Autodesk Inventor part; units mm, degrees
ref_plane "YZ Plane" through (0, 0, 0) normal (1, 0, 0) x (0, 1, 0)
ref_plane "XZ Plane" through (0, 0, 0) normal (0, 1, 0) x (-1, 0, 0)
ref_plane "XY Plane" through (0, 0, 0) normal (0, 0, 1) x (1, 0, 0)
sketch "Sketch1" plane through (0, 0, 0) normal (0, 1, 0) x (-1, 0, 0)
  point P0 (0, 0)
sketch "Sketch2" plane through (0, 0, 0) normal (0, 1, 0) x (-1, 0, 0)
  line L0 (68, -12) -> (68, -66)
  line L1 (68, -66) -> (0, -66)
  line L2 (0, -66) -> (0, -12)
  line L3 (68, -12) -> (0, -12)
  point P0 (0, 0)
  dimension "d0" = 68
  dimension "d138" = 54
extrude "Extrusion1" add sketch "Sketch2" along normal blind 17.5
sketch "Sketch3" plane through (0, 17.5, 0) normal (0, 1, 0) x (1, 0, 0)
  line L0 (0, 66) -> (-68, 66)
  line L1 (-68, 66) -> (0, 66)
  line L2 (-68, 66) -> (0, 66)
  line L3 (0, 66) -> (-68, 66)
  line L4 (-68, 66) -> (-68, 12)
  line L5 (-68, 12) -> (0, 12)
  line L6 (0, 66) -> (0, 12)
  dimension "d135" = 68
  dimension "d136" = 54
sketch "Sketch4" plane through (0, 17.5, 0) normal (0, 1, 0) x (1, 0, 0)
  line L0 (0, 66) -> (-68, 66)
  line L1 (-30.4814, 66) -> (-28.4814, 66)
  line L2 (-28.4814, 66) -> (-28.4814, 64)
  line L3 (-68, 66) -> (-68, 12)
  line L4 (-68, 37.8423) -> (-68, 39.8423)
  line L5 (-68, 39.8423) -> (-66, 39.8423)
  line L6 (0, 38.8423) -> (0, 36.8423)
  line L7 (0, 36.8423) -> (-2, 36.8423)
  line L8 (-66, 64) -> (-2, 64)
  line L9 (-2, 64) -> (-2, 14)
  line L10 (-2, 14) -> (-66, 14)
  line L11 (-66, 14) -> (-66, 64)
  dimension "d5" = 2
  dimension "d6" = 2
  dimension "d7" = 2
  dimension "d11" = 2
  dimension "d75" = 2
  dimension "d132" = 50
  dimension "d133" = 64
extrude "Extrusion2" cut sketch "Sketch4" against normal blind 15.5 contours L8 L9 L10 L11
sketch "Sketch7" plane through (0, 17.5, 0) normal (0, 1, 0) x (1, 0, 0)
  line L0 (-68, 66) -> (-67, 66)
  line L1 (-68, 66) -> (-6, 66)
  line L2 (-68, 65) -> (-68, 66)
  line L3 (0, 66) -> (-7, 66)
  line L4 (-67, 65) -> (-1, 65)
  line L5 (0, 66) -> (-68, 66)
  line L6 (-68, 66) -> (0, 66)
  line L7 (0, 12) -> (0, 66)
  line L8 (0, 12) -> (-1, 12)
  line L9 (-1, 66) -> (0, 66)
  line L10 (0, 66) -> (0, 12)
  line L11 (0, 12) -> (-1, 12)
  line L12 (-68, 12) -> (0, 12)
  line L13 (-1, 65) -> (-1, 12)
  line L14 (0, 12) -> (-1, 12)
  line L15 (-67, 65) -> (-67, 12)
  line L16 (-68, 66) -> (-68, 12)
  line L17 (-67, 12) -> (-68, 12)
  line L18 (-68, 12) -> (-68, 66)
  dimension "d76" = 1
  dimension "d139" = 1
  dimension "d140" = 1
extrude "Extrusion3" cut sketch "Sketch7" against normal blind 2 contours L0 L1 L3 L7 L8 L13 L4 L15 L12 L16 L2
sketch "Sketch8" plane through (0, 17.5, 0) normal (0, 1, 0) x (1, 0, 0)
  line L0 (0, 12) -> (0, 13)
  line L1 (0, 13) -> (-68, 13)
  line L2 (0, 12) -> (-68, 12)
  line L3 (-68, 12) -> (-68, 13)
  line L4 (-67, 12) -> (-1, 12)
  point P0 (0, 0)
  point P1 (-70, 0)
  dimension "d46" = 68
  dimension "d141" = 1
extrude "Extrusion4" cut sketch "Sketch8" against normal blind 2
sketch "Sketch10" plane through (0, 2, 0) normal (0, 1, 0) x (1, 0, 0)
  line L0 (-31, 2) -> (-41, 2)
  line L1 (-63, 64) -> (-48, 64)
  line L2 (-48, 64) -> (-48, 61)
  line L3 (-48, 61) -> (-63, 61)
  line L4 (-63, 61) -> (-63, 64)
  line L5 (-22, 14) -> (-7, 14)
  line L6 (-7, 14) -> (-7, 17)
  line L7 (-7, 17) -> (-22, 17)
  line L8 (-22, 17) -> (-22, 14)
  line L9 (-66, 14) -> (-66, 64)
  line L10 (-2, 14) -> (-66, 14)
  line L11 (-66, 64) -> (-2, 64)
  line L12 (-2, 64) -> (-2, 14)
  line L13 (-2, 14) -> (-66, 14)
  line L14 (-66, 14) -> (-66, 64)
  point P0 (0, 0)
  point P1 (-21, 64)
  dimension "d57" = 15
  dimension "d58" = 3
  dimension "d61" = 15
  dimension "d79" = 3
extrude "Extrusion5" add sketch "Sketch10" along normal blind 18 contours L1 L2 L3 L4 | L8 L7 L6 L5
sketch "Sketch11" plane through (0, 0, 0) normal (0, -1, 0) x (1, 0, 0)
  circle A0 centre (-12, -42.73) radius 4
  circle A1 centre (-33.5, -54.23) radius 1.5
  line L0 (0, 0) -> (0, -66)
  line L1 (0, -66) -> (-68, -66)
  line L2 (-2, -64) -> (-2, -14)
  dimension "d85" = 23.27
  dimension "d86" = 21.5
  dimension "d88" = 8
  dimension "d89" = 3
  dimension "d119" = 11.5
  dimension "d120" = 10
extrude "Extrusion6" cut sketch "Sketch11" against normal blind 9
sketch "Sketch12" plane through (0, 0, 0) normal (0, -1, 0) x (1, 0, 0)
  line L0 (-68, -12) -> (-68, -66)
  line L1 (0, -12) -> (0, -6)
  line L2 (0, -6) -> (-68, -6)
  line L3 (-68, -6) -> (-68, -12)
  line L4 (-68, -12) -> (0, -12)
  line L5 (0, -12) -> (-68, -12)
  point P0 (0, 0)
  point P1 (-70, 0)
  dimension "d81" = 6
  dimension "d143" = 68
  dimension "d144" = 0
extrude "Extrusion7" add sketch "Sketch12" against normal blind 29.5
sketch "Sketch15" plane through (0, 0, -66) normal (1, 0, 0) x (0, 0, -1)
  line L0 (-27.77, 17.5) -> (-18.77, 17.5)
  line L1 (-18.77, 17.5) -> (-18.77, 12.5)
  line L2 (-18.77, 12.5) -> (-27.77, 12.5)
  line L3 (-27.77, 12.5) -> (-27.77, 17.5)
  line L4 (-54, 0) -> (-54, 29.5)
  line L5 (0, 0) -> (0, 15.5)
  line L6 (0, 0) -> (-60, 0)
  line L7 (0, 15.5) -> (-54, 15.5)
  line L8 (-23.27, -7.8454) -> (-23.27, 0)
  line L9 (-23.27, 0) -> (-23.27, 15.5)
  point P0 (-66, 0)
  point P1 (-66, 14.75)
  point P2 (0, 16.75)
  dimension "d108" = 9
  dimension "d109" = 5
  dimension "d111" = 27.77
extrude "Extrusion9" cut sketch "Sketch15" against normal blind 10 contours L0 L1 L7 L3 | L7 L9 L2 L3 | L1 L2 L9 L7
fillet "Fillet7" radius 2 1 edges at (0, 7.75, -66)
fillet "Fillet8" radius 2 1 edges at (-68, 7.75, -66)
fillet "Fillet9" radius 2 1 edges at (0, 14.75, -6)
fillet "Fillet11" radius 2 1 edges at (-68, 14.75, -6)
sketch "Sketch16" plane through (-2, 0, -6) normal (0, 0, 1) x (1, 0, 0)
  line L0 (2, 29.5) -> (-66, 29.5)
  line L1 (-32, 29.5) -> (-32, 0)
  line L2 (-46, 2) -> (0, 2)
  line L3 (-66, 0) -> (-66, 15.5)
  line L4 (-66, 15.5) -> (-66, 29.5)
  line L5 (-32, 14.75) -> (-64, 14.75)
  line L6 (-64, 0) -> (-64, 29.5)
  circle A0 centre (-32, 14.75) radius 2.5
  point P0 (2, 0)
  dimension "d148" = 5
extrude "Extrusion10" cut sketch "Sketch16" against normal blind 6 contours A0 L1 | L1 L5 A0 | L1 A0 L5
sketch "Sketch17" plane through (-2, 0, -66) normal (0, 0, -1) x (-1, 0, 0)
  line L0 (3, 20.5) -> (11.5, 20.5)
  line L1 (11.5, 20.5) -> (11.5, 15.5)
  line L2 (11.5, 15.5) -> (3, 15.5)
  line L3 (3, 15.5) -> (3, 20.5)
  line L4 (18.1, 20.5) -> (26.6, 20.5)
  line L5 (26.6, 20.5) -> (26.6, 15.5)
  line L6 (26.6, 15.5) -> (18.1, 15.5)
  line L7 (18.1, 15.5) -> (18.1, 20.5)
  line L8 (66, 0) -> (66, 15.5)
  line L9 (-1, 17.5) -> (65, 17.5)
  line L10 (64, 15.5) -> (0, 15.5)
  line L11 (-2, 15.5) -> (-2, 0)
  dimension "d151" = 8.5
  dimension "d152" = 8.5
  dimension "d153" = 5
  dimension "d157" = 0
  dimension "d158" = 13.5
  dimension "d160" = 28.6
extrude "Extrusion11" cut sketch "Sketch17" against normal blind 10 contours L0 L1 L9 L3 | L9 L1 L2 L3 | L9 L5 L6 L7 | L7 L4 L5 L9
properties part number "Shell 3 top"
Here's how the part is built. I have some questions about the finished solid (model axes, mm). A direction names the side the tool comes from. Round coordinates to 2 decimals unless told otherwise and drop trailing zeros. Order: outer loops, then holes, each group sorted by start corner. A loop starts at its lowest first (then second) coordinate and runs counter-clockwise, first axis right, second up. Notation, with made-up numbers: (-34.75, 35.25) -> (15.25, 35.25) arc R23 cw to (15.25, 48.25) -> close; hole circle Ø1 at (37.25, 54). An arc over 180 degrees is marked (long way). Use a Markdown table: item, result. Add a question column.
(1) Suppose I cut it at A-A, the plane z = -42.73. Please give me the cut outline in (x, y).
(2) Suppose I cut it at C-C, the plane y = 8. Please give me the cut outline in (x, z), and give its area (3 significant figures).
(3) If we mould it in two halves opening along Z, with no side actions, what happens to faces 1 (the face through (-48, 17, -65)), 2 (the face through (-63, 11, -62)), 3 (the face through (-56, 20, -63))? For each: released by +Z, released by -Z, zero draft, split by the parting line, or undercut.
(4) Suppose I cut it at D-D, the plane z = -62. Please give me the cut outline in (x, y), and give its area (3 significant figures).
(5) For pin 1 Ø1.5 at (x, z) = (-58.5, -63) entering from +Y; pin 2 Ø1 at (y, z) = (18.5, -27.5) entering from -X; pin 3 Ø4 at (x, z) = (-57.5, -15) entering from +Y; pin 4 Ø1.1 at (y, z) = (16.5, -64.5) entering from -X, each with a flat end and sliding along its axis, tell me the tip position at first contact or that it passes through.
(6) Suppose I cut it at B-B, the plane x = -12. Please give me the cut outline in (y, z), and give its area (3 significant figures).
(7) I need wall thicknesses on line 1 along X through (y, z) = (8, -14.5); line 2 along Z through (x, y) = (-10.5, 7.5); line 3 along X through (y, z) = (9.5, -62). Which ranges of each line are inside material? Lowest first, please.
(8) For faces 4 (the face through (-1, 12.5, -43)), 5 (the face through (-25, 10, -64)), 6 (the face through (-1.8, 17.5, -56.7)), 7 (the face through (-56, 19, -64)), which set-ups out of +Z, -Z, +X, -X, +Y, -Y let a thin tool reach every point of the face, with its end or its side?
Verdict:
| question | item | result |
|---|---|---|
| 1 | outline | (-68, 0) -> (-16, 0) -> (-16, 2) -> (-66, 2) -> (-66, 17.5) -> (-67, 17.5) -> (-67, 15.5) -> (-68, 15.5) -> close; (-8, 0) -> (0, 0) -> (0, 12.5) -> (-2, 12.5) -> (-2, 2) -> (-8, 2) -> close |
| 2 | outline | (-68, -64) arc R2 ccw to (-66, -66) -> (-2, -66) arc R2 ccw to (0, -64) -> (0, -8) arc R2 ccw to (-2, -6) -> (-66, -6) arc R2 ccw to (-68, -8) -> close; hole (-66, -64) -> (-63, -64) -> (-63, -61) -> (-48, -61) -> (-48, -64) -> (-2, -64) -> (-2, -14) -> (-7, -14) -> (-7, -17) -> (-22, -17) -> (-22, -14) -> (-66, -14) -> close |
| 2 | area | 967 mm2 |
| 3 | face 1 | released by -Z |
| 3 | face 2 | undercut |
| 3 | face 3 | zero draft |
| 4 | outline | (-68, 0) -> (0, 0) -> (0, 15.5) -> (-1, 15.5) -> (-1, 17.5) -> (-2, 17.5) -> (-2, 2) -> (-48, 2) -> (-48, 20) -> (-63, 20) -> (-63, 2) -> (-66, 2) -> (-66, 17.5) -> (-67, 17.5) -> (-67, 15.5) -> (-68, 15.5) -> close |
| 4 | area | 464 mm2 |
| 5 | pin 1 | y = 20 |
| 5 | pin 2 | through |
| 5 | pin 3 | y = 17.5 |
| 5 | pin 4 | x = -67 |
| 6 | outline | (0, -66) -> (15.5, -66) -> (15.5, -64) -> (2, -64) -> (2, -46.73) -> (0, -46.73) -> close; (0, -38.73) -> (2, -38.73) -> (2, -17) -> (20, -17) -> (20, -14) -> (17.5, -14) -> (17.5, -13) -> (15.5, -13) -> (15.5, -12) -> (29.5, -12) -> (29.5, -6) -> (0, -6) -> close |
| 6 | area | 379 mm2 |
| 7 | line 1 | -68 to -66, -22 to -7, -2 to 0 |
| 7 | line 2 | -66 to -64, -17 to -6 |
| 7 | line 3 | -68 to -66, -63 to -48, -2 to 0 |
| 8 | face 4 | +X, +Y |
| 8 | face 5 | +Y |
| 8 | face 6 | -Z, +X, +Y |
| 8 | face 7 | -Z, +X, -X, +Y |
